Here's how the part is built. I have some questions about the finished solid (model axes, mm). Face numbers are marked on the shaded views. Round coordinates to 2 decimals unless told otherwise and drop trailing zeros. Order: outer loops, then holes, each group sorted by start corner. A loop starts at its lowest first (then second) coordinate and runs counter-clockwise, first axis right, second up. Notation, with made-up numbers: (-35, 8.5) -> (-29, 8.5) arc R37 cw to (-29, 46.5) -> close; hole circle Ø6 at (1.5, 7). An arc over 180 degrees is marked (long way). Use a Markdown table: item, result. Add a question column.
(1) I want a section at D-D, the plane y = 167.5. Please give me the cut outline in (x, z), then the cut area to 3 significant figures.
(2) I want a section at A-A, the plane z = 0. Please give me the cut outline in (x, y) (1 decimal), then the cut area to 3 significant figures.
(3) I want a section at B-B, the plane x = 0. Please give me the cut outline in (y, z) (1 decimal), then the cut area to 3 significant figures.
(4) Thinking about a two-plate mould opening in X: for the marked faces 1, 2 and 3, which applies, pulls with the +X half, pulls with the -X half, needs draft (parallel to the pull), parting line crosses it, or undercut?
(5) I want a section at C-C, the plane y = 208. Please give me the cut outline in (x, z), then the cut area to 3 significant figures.
(6) I'm going to push flat-ended pins straight in: P1, Ø10, axis at y = 168.5, z = -65, coming from the -X side; P2, Ø12, axis at x = -66.5, y = 186, coming from the +Z side; P3, Ø8, axis at y = 179, z = -45.5, coming from the -X side. Where does each tip first touch, or does it pass through?
(7) If I drill on probe 1 along Y at (x, z) = (18, -21) (3 decimals); probe 2 along Z at (x, y) = (46, 224); probe 3 along Z at (x, y) = (-86.5, 179), over which ranges is the centre line in solid material (lowest first)?
from build123d import *


with BuildPart() as part:
    # Sketch1 → Revolve1 (revolve)
    with BuildSketch(Plane.XY):
        with BuildLine():
            Line((0, 0), (66.209470016, 0))
            ThreePointArc((66.209470016, 0), (73.862659994, 2.785533349), (77.934837326, 9.838751385))
            Line((77.934837326, 9.838751385), (116.50834779, 228.6))
            ThreePointArc((116.50834779, 228.6), (112.127650699, 233.380691976), (106.98334779, 229.43332952))
            Line((106.98334779, 229.43332952), (68.554543478, 11.492750277))
            ThreePointArc((68.554543478, 11.492750277), (67.740108012, 10.08210667), (66.209470016, 9.525))
            Line((66.209470016, 9.525), (0, 9.525))
            Line((0, 9.525), (0, 0))
        make_face()
    revolve(axis=Axis((0, 0, 0), (0, 1, 0)))


solid = part.part
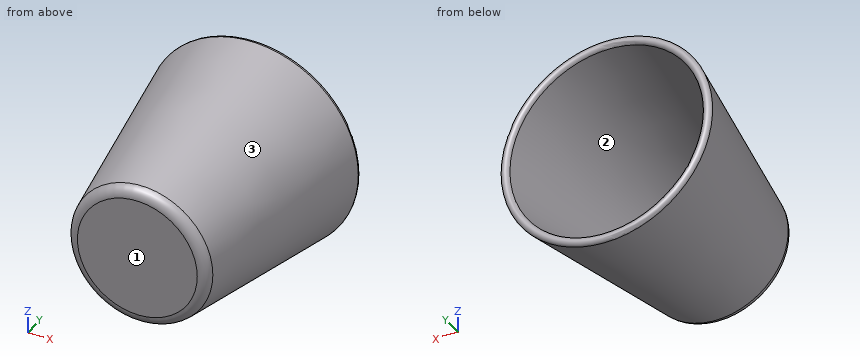
Taken from the geometry:
| question | item | result |
|---|---|---|
| 1 | outline | circle Ø211.47 at (0, 0); hole circle Ø192.13 at (0, 0) |
| 1 | area | 6,130 mm2 |
| 2 | outline | (-116.5, 228.6) -> (-77.9, 9.8) arc R11.9 ccw to (-66.2, 0) -> (66.2, 0) arc R11.9 ccw to (77.9, 9.8) -> (116.5, 228.6) arc R4.8 ccw to (107, 229.4) -> (68.6, 11.5) arc R2.4 cw to (66.2, 9.5) -> (-66.2, 9.5) arc R2.4 cw to (-68.6, 11.5) -> (-107, 229.4) arc R4.8 ccw to start |
| 2 | area | 5,740 mm2 |
| 3 | outline | (0, -66.2) arc R11.9 ccw to (9.8, -77.9) -> (228.6, -116.5) arc R4.8 ccw to (229.4, -107) -> (11.5, -68.6) arc R2.4 cw to (9.5, -66.2) -> (9.5, 66.2) arc R2.4 cw to (11.5, 68.6) -> (229.4, 107) arc R4.8 ccw to (228.6, 116.5) -> (9.8, 77.9) arc R11.9 ccw to (0, 66.2) -> close |
| 3 | area | 5,740 mm2 |
| 4 | face 1 | needs draft |
| 4 | face 2 | undercut |
| 4 | face 3 | parting line crosses it |
| 5 | outline | circle Ø225.75 at (0, 0); hole circle Ø206.41 at (0, 0) |
| 5 | area | 6,570 mm2 |
| 6 | P1 | stops at x = -87.44 |
| 6 | P2 | stops at z = 90.86 |
| 6 | P3 | stops at x = -99.62 |
| 7 | probe 1 | y = 0 to 9.525 |
| 7 | probe 2 | z = -106.16 to -95.53, 95.53 to 106.16 |
| 7 | probe 3 | z = -64.27 to -46.25, 46.25 to 64.27 |
